Source: CAD feature listing. Evaluate the final solid. Frame: model axes, mm. Face numbers are marked on the shaded views. A direction names the side the tool comes from. Round coordinates to 2 decimals unless told otherwise and drop trailing zeros. Loops run counter-clockwise (first coordinate to the right, second up) from the corner with the lowest first, then second, coordinate; pieces in that order, holes last. Notation, with made-up numbers: (78.5, 9.5) -> (93.5, 9.5) arc R5 ccw to (93.5, 15.5) -> close; hole circle Ø5 at (-21, 26). An arc over 180 degrees is marked (long way). Return JSON: item names as keys, results as strings. Group by question number.
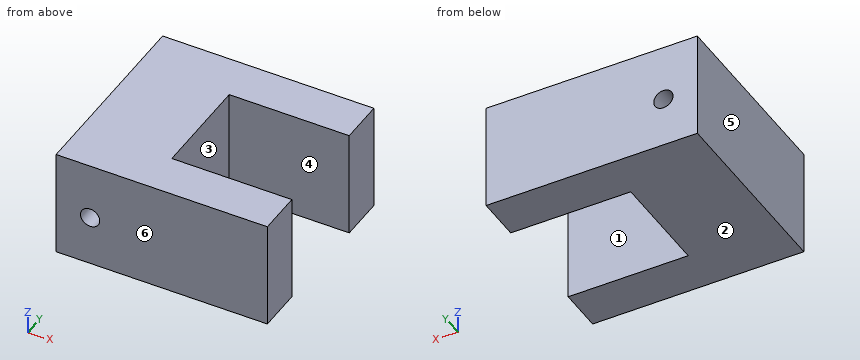
```python
from build123d import *

# Parameters (mm, degrees)
IZIM1_W                     = 88
IZIM1_H                     = 80
Y_KSEKLIK_EKSTR_ZYON1_DEPTH = 45
IZIM2_W                     = 50
IZIM2_H                     = 43.119063511
KES_EKSTR_ZYON1_DEPTH       = 75.57211275
IZIM3_R                     = 4.00297174
KES_EKSTR_ZYON2_DEPTH       = 102.788997441


with BuildPart() as part:
    # Çizim1 → Yükseklik-Ekstrüzyon1 (new body)
    with BuildSketch(Plane.XY):
        Rectangle(IZIM1_W, IZIM1_H)
    extrude(amount=Y_KSEKLIK_EKSTR_ZYON1_DEPTH)

    # Çizim2 → Kes-Ekstrüzyon1 (cut, through all)
    with BuildSketch(Plane.XY.offset(45)):
        with Locations((19, -0.059531756)):
            Rectangle(IZIM2_W, IZIM2_H)
    extrude(amount=-KES_EKSTR_ZYON1_DEPTH, mode=Mode.SUBTRACT)

    # Çizim3 → Kes-Ekstrüzyon2 (cut, through all)
    with BuildSketch(Plane(origin=(0, 40, 0), x_dir=(1, 0, 0), z_dir=(0, 1, 0))):
        with Locations(Location((-29.85, -21.15, 0), (0, 0, 270))):
            Circle(IZIM3_R)
    extrude(amount=-KES_EKSTR_ZYON2_DEPTH, mode=Mode.SUBTRACT)


solid = part.part
```
(1) Cut plane B-B (z = 21.15). Return loops of the section in (x, y), and give its area (3 significant figures).
(2) Cut plane C-C (z = 10). Return loops of the section in (x, y).
(3) Set-up query: the marked faces 1 and 2. Return all of +Z, -Z, +X, -X, +Y, -Y with unobstructed straight access to the full face (end or side cutting, diameter ignored); none if empty.
(4) Cut plane A-A (x = -29.85). Return loops of the section in (y, z).
(5) Cut plane D-D (x = 29.5). Return loops of the section in (y, z), and give its area (3 significant figures).
(6) Ray query, line 1 (X direction, y = -10.5, z = 21.15); line 2 (Y direction, x = 7, z = 15); line 3 (X direction, y = -20, z = 36). Return the intervals inside material, ascending.
(7) Pin query (flat end, axial travel): pin 1 (6 mm diameter, centred on y = 7, z = 11.5, fed in from +X). Return the tip coordinate at first contact, or that it passes through.
(8) Mould query, pull axis Y, two halves, no side actions, for the marked faces 3, 4, 5 and 6. Classes: released by +Y, released by -Y, zero draft, split by the parting line, or undercut.
Answers follow:
{
 "1": {"outline": "(-44, -40) -> (-33.85, -40) -> (-33.85, 40) -> (-44, 40) -> close; (-25.85, -40) -> (44, -40) -> (44, -21.62) -> (-6, -21.62) -> (-6, 21.5) -> (44, 21.5) -> (44, 40) -> (-25.85, 40) -> close", "area": "4,240 mm^2"},
 "2": {"outline": "(-44, -40) -> (44, -40) -> (44, -21.62) -> (-6, -21.62) -> (-6, 21.5) -> (44, 21.5) -> (44, 40) -> (-44, 40) -> close"},
 "3": {"face 1": "+Z, -Z, +X", "face 2": "-Z, +X, -X, +Y, -Y"},
 "4": {"outline": "(-40, 0) -> (40, 0) -> (40, 17.15) -> (-40, 17.15) -> close; (-40, 25.15) -> (40, 25.15) -> (40, 45) -> (-40, 45) -> close"},
 "5": {"outline": "(-40, 0) -> (-21.62, 0) -> (-21.62, 45) -> (-40, 45) -> close; (21.5, 0) -> (40, 0) -> (40, 45) -> (21.5, 45) -> close", "area": "1,660 mm^2"},
 "6": {"line 1": "-44 to -33.85, -25.85 to -6", "line 2": "-40 to -21.62, 21.5 to 40", "line 3": "-44 to -6"},
 "7": {"pin 1": "x = -6"},
 "8": {"face 3": "undercut", "face 4": "undercut", "face 5": "zero draft", "face 6": "released by -Y"}
}
